Could you check a few things on this model? Use its own coordinates, in mm. A direction names the side the tool comes from. Round coordinates to 2 decimals unless told otherwise and drop trailing zeros. Loops run counter-clockwise (first coordinate to the right, second up) from the corner with the lowest first, then second, coordinate; pieces in that order, holes last. Notation, with made-up numbers: (-20, 42) -> (13, 42) arc R15 ccw to (13, 53) -> close; hole circle Ø6 at (12.25, 32). An arc over 180 degrees is marked (long way). Write each question's results on one line, items separated by ' | '.
Autodesk Inventor part; units mm, degrees
ref_plane "YZ Plane" through (0, 0, 0) normal (1, 0, 0) x (0, 1, 0)
ref_plane "XZ Plane" through (0, 0, 0) normal (0, 1, 0) x (-1, 0, 0)
ref_plane "XY Plane" through (0, 0, 0) normal (0, 0, 1) x (1, 0, 0)
sketch "Sketch1" plane through (0, 0, 0) normal (0, 1, 0) x (-1, 0, 0)
  line L0 (0, 0) -> (25.4, 0)
  line L1 (25.4, 0) -> (25.4, -38.1)
  line L2 (25.4, -38.1) -> (0, -38.1)
  line L3 (0, -38.1) -> (0, 0)
  circle A0 centre (12.7, -6.35) radius 2.4892
  circle A1 centre (12.7, -19.05) radius 2.4892
  circle A2 centre (12.7, -31.75) radius 2.4892
  point P0 (12.7, -38.1)
  dimension "d1" = 38.1
  dimension "d2" = 25.4
  dimension "d3" = 4.9784
  dimension "d4" = 6.35
  dimension "d7" = 12.7
extrude "Extrusion1" add sketch "Sketch1" along normal blind 6.35
sketch "Sketch2" plane through (0, 6.35, 0) normal (0, 1, 0) x (1, 0, 0)
  line L0 (0, 38.1) -> (-25.4, 38.1)
  line L1 (0, 38.1) -> (-6.35, 38.1)
  line L2 (-6.35, 38.1) -> (-6.35, 0)
  line L3 (-6.35, 0) -> (0, 0)
  line L4 (0, 0) -> (0, 38.1)
  point P0 (0, 0)
  dimension "d14" = 6.35
  dimension "d15" = 38.1
extrude "Extrusion2" add sketch "Sketch2" along normal blind 30.48
sketch "Sketch3" plane through (0, 0, 0) normal (1, 0, 0) x (0, 0, -1)
  line L0 (0, 6.35) -> (0, 36.83)
  line L1 (0, 36.83) -> (15.875, 36.8288)
  line L2 (38.1, 6.35) -> (38.1, 36.83)
  line L3 (38.1, 36.83) -> (22.225, 36.83)
  line L4 (38.1, 36.83) -> (0, 36.83)
  line L5 (22.225, 36.83) -> (15.8731, 36.83)
  line L6 (15.8731, 36.83) -> (15.8731, 11.9339)
  line L7 (22.225, 11.9339) -> (22.225, 36.83)
  arc A0 (15.8731, 11.9339) -> (22.225, 11.9339) centre (19.049, 11.9339) ccw
  point P0 (0, 0)
  dimension "d18" = 15.875
  dimension "d19" = 15.875
extrude "Extrusion3" cut sketch "Sketch3" against normal blind 30.48
properties part number "BUMPER BRACKETS" material "Aluminum 6061"
1) I want a section at D-D, the plane y = 13. Write out the boundary of the cut face in (x, z) (3 decimals), plus the area to 3 significant figures.
Model answer:
outline: (-6.35, -38.1) -> (0, -38.1) -> (0, -22.225) -> (-6.35, -22.225) -> close; (-6.35, -15.873) -> (0, -15.873) -> (0, 0) -> (-6.35, 0) -> close | area: 202 mm2
2) I want a section at C-C, the plane x = -12.7. Write out the boundary of the cut face in (y, z).
Model answer:
outline: (0, -38.1) -> (6.35, -38.1) -> (6.35, -34.24) -> (0, -34.24) -> close; (0, -29.26) -> (6.35, -29.26) -> (6.35, -21.54) -> (0, -21.54) -> close; (0, -16.56) -> (6.35, -16.56) -> (6.35, -8.84) -> (0, -8.84) -> close; (0, -3.86) -> (6.35, -3.86) -> (6.35, 0) -> (0, 0) -> close
3) I want a section at A-A, the plane z = -19.05. Write out the boundary of the cut face in (x, y), plus the area to 3 significant figures.
Model answer:
outline: (-25.4, 0) -> (-15.19, 0) -> (-15.19, 6.35) -> (-25.4, 6.35) -> close; (-10.21, 0) -> (0, 0) -> (0, 8.76) -> (-6.35, 8.76) -> (-6.35, 6.35) -> (-10.21, 6.35) -> close | area: 145 mm2
4) I want a section at B-B, the plane y = 5. Write out the boundary of the cut face in (x, z), plus the area to 3 significant figures.
Model answer:
outline: (-25.4, -38.1) -> (0, -38.1) -> (0, 0) -> (-25.4, 0) -> close; hole circle Ø4.98 at (-12.7, -31.75); hole circle Ø4.98 at (-12.7, -19.05); hole circle Ø4.98 at (-12.7, -6.35) | area: 909 mm2
5) I need wall thicknesses on line 1 (Z direction, x = -12.7, y = 4.75); line 2 (Y direction, x = -19, z = -32); line 3 (X direction, y = 22, z = -24). Which ranges of each line are inside material? Lowest first, please.
Model answer:
line 1: z = -38.1 to -34.24, -29.26 to -21.54, -16.56 to -8.84, -3.86 to 0 | line 2: y = 0 to 6.35 | line 3: x = -6.35 to 0
6) I'm going to push flat-ended pins straight in: pin 1 (4 mm diameter, centred on x = -12.7, z = -19.05, fed in from -Y); pin 2 (15 mm diameter, centred on x = -18, z = -25, fed in from +Y); pin 3 (9 mm diameter, centred on y = 27, z = -19, fed in from -X). Where does each tip first touch, or does it pass through?
Model answer:
pin 1: passes through | pin 2: stops at y = 6.35 | pin 3: stops at x = -6.35
7) For faces 1 (the flat face through (-16, 6.35, -19)), 2 (the flat face through (-3, 24, -22.225)), 3 (the cylindrical face through (-10.213, 3.131, -31.859)), which set-ups out of +Z, -Z, +X, -X, +Y, -Y let a thin tool reach every point of the face, with its end or its side?
Model answer:
face 1: +Z, -Z, -X, +Y | face 2: +X, -X, +Y | face 3: +Y, -Y
